Work out the finished part from the listing and answer in its coordinate system (mm). A direction names the side the tool comes from. Round coordinates to 2 decimals unless told otherwise and drop trailing zeros. Order: outer loops, then holes, each group sorted by start corner. A loop starts at its lowest first (then second) coordinate and runs counter-clockwise, first axis right, second up. Notation, with made-up numbers: (51, -22.5) - (95, -22.5) arc R15 cw to (95, -1.5) - close; hole circle Ø1 at (-23, 24.25). An arc over 180 degrees is marked (long way). Put each result on its own line as item: value.
```python
from build123d import *

# Parameters (mm, degrees)
F1_DEPTH = 125
F3_DEPTH = 149.2
F4_W     = 2
F4_H     = 5.5
F5_DEPTH = 1.201
F4_W_2   = 1.2
F4_H_2   = 7.7
F6_DEPTH = 5.5
F7_R     = 1.95
F8_R     = 1.95
F9_DEPTH = 78.4


with BuildPart() as f1:
    # F0 (on Right) → F1 (new body, symmetric)
    with BuildSketch(Plane.YZ):
        Polygon((0, 148), (0, 0), (1.2, 0), (1.2, 149.2), (-30.2, 149.2), (-30.2, 105.6), (-29, 105.6), (-29, 148), align=None)
    extrude(amount=F1_DEPTH, both=True)

    # F2 (on face) → F3 (join, through all)
    with BuildSketch(Plane(origin=(0, 0, 0), x_dir=(1, 0, 0), z_dir=(0, 0, -1))):
        Polygon((125, 29), (125, -1.2), (126.2, -1.2), (126.2, 30.2), (115, 30.2), (115, 29), align=None)
    extrude(amount=-F3_DEPTH)

    # F4 (on face) → F5 (cut, through all)
    with BuildSketch(Plane.XZ):
        with Locations((23.375, 104.75)):
            Rectangle(F4_W, F4_H)
        with Locations((106.625, 104.75)):
            Rectangle(F4_W, F4_H)
        with Locations((11.625, 93.45)):
            Rectangle(F4_W, F4_H)
        with Locations((-71.625, 93.45)):
            Rectangle(F4_W, F4_H)
    extrude(amount=-F5_DEPTH, mode=Mode.SUBTRACT)

    # F4 (on face) → F6 (join)
    with BuildSketch(Plane.XZ):
        with Locations((26.4, 22)):
            Rectangle(F4_W_2, F4_H_2)
        with Locations((103.6, 22)):
            Rectangle(F4_W_2, F4_H_2)
        with Locations((-68.6, 10.7)):
            Rectangle(F4_W_2, F4_H_2)
        with Locations((8.6, 10.7)):
            Rectangle(F4_W_2, F4_H_2)
    extrude(amount=F6_DEPTH)

    # F7 (on face) + F8 (on face) → F9 (cut, through all)
    with BuildSketch(Plane(origin=(25.8, 0, 0), x_dir=(0, -1, 0), z_dir=(-1, 0, 0))):
        with Locations((2.75, 22)):
            Circle(F7_R)
    with BuildSketch(Plane(origin=(-69.2, 0, 0), x_dir=(0, -1, 0), z_dir=(-1, 0, 0))):
        with Locations((2.75, 10.7)):
            Circle(F8_R)
    extrude(amount=-F9_DEPTH, mode=Mode.SUBTRACT)


solid = f1.part
```
1) A cutting plane is placed at B-B on x = -78.5. Write down the section's boundary in (y, z), then the cut area to 3 significant figures.
Findings below:
outline: (-30.2, 105.6) - (-29, 105.6) - (-29, 148) - (0, 148) - (0, 0) - (1.2, 0) - (1.2, 149.2) - (-30.2, 149.2) - close
area: 266 mm2
2) A cutting plane is placed at C-C on y = -8. Write down the section's boundary in (x, z).
Findings below:
outline: (-125, 148) - (125, 148) - (125, 0) - (126.2, 0) - (126.2, 149.2) - (-125, 149.2) - close
3) A cutting plane is placed at A-A on z = 66. Write down the section's boundary in (x, y), then the cut area to 3 significant figures.
Findings below:
outline: (-125, 0) - (125, 0) - (125, -29) - (115, -29) - (115, -30.2) - (126.2, -30.2) - (126.2, 1.2) - (-125, 1.2) - close
area: 350 mm2
4) Straight lines are drawn through the part: L1, parallel to Z at x = 103.7, y = -2.75; L2, parallel to X at y = -2.5, z = 14; L3, parallel to Z at x = -68.35, y = -2.75. For each, find the intervals that lie inside material, in ascending order. Write a range as from..to.
Findings below:
L1: z = 18.15..20.05, 23.95..25.85, 148..149.2
L2: x = -69.2..-68, 8..9.2, 125..126.2
L3: z = 6.85..8.75, 12.65..14.55, 148..149.2
5) For a pull along X with two mould halves and no side action, classify faces 4 (the flat face through (8, -5, 10)), 5 (the flat face through (-125, 1, 86)), 6 (the flat face through (-1, 1.2, 74)) as pulls with the +X half, pulls with the -X half, needs draft (parallel to the pull), parting line crosses it, or undercut.
Findings below:
face 4: undercut
face 5: pulls with the -X half
face 6: needs draft
6) For faces 1 (the flat face through (19, -29, 123)), 2 (the flat face through (25.8, -5, 23)), 3 (the flat face through (-68, -5, 10)), determine the directions among +Z, -Z, +X, -X, +Y, -Y from which every point of the face is accessible in a straight line to the end or side of a thin tool.
Findings below:
face 1: -Z, -X
face 2: -Z, -X, -Y
face 3: -Z, -Y
7) Given pin 1 Ø0.6 at (x, y) = (-61.5, -29.5) entering from -Z; pin 2 Ø0.6 at (x, z) = (26.5, 22) entering from -Y; pin 3 Ø10 at (x, z) = (-46.5, 91.5) entering from -Y, each flat-ended and moving along its own axis, determine where each tip first touches the part or whether it passes through.
Findings below:
pin 1: stops at z = 105.6
pin 2: stops at y = -5.5
pin 3: stops at y = 0
